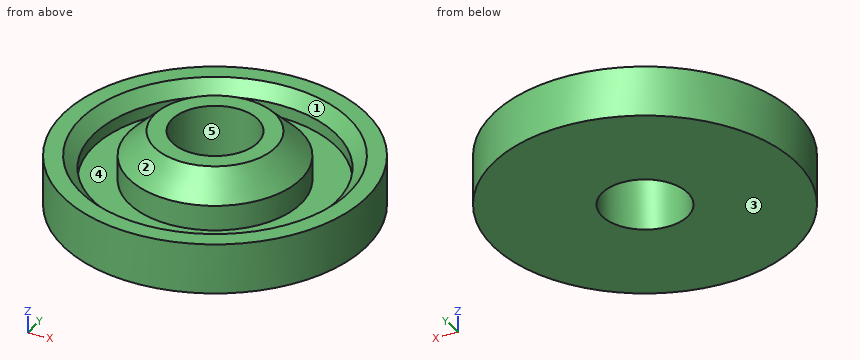
```python
from build123d import *

# Parameters (mm, degrees)
SKETCH2_R          = 1.6933
CUT_EXTRUDE1_DEPTH = 10


with BuildPart() as part:
    # Sketch1 → Revolve1 (revolve)
    with BuildSketch(Plane(origin=(0, 0, 0), x_dir=(1, 0, 0), z_dir=(0, 1, 0)), mode=Mode.PRIVATE) as revolve1_sk:
        Polygon((0, 0), (6, 0), (6, -2), (5.3, -2), (4.8, -1.5), (4.8, -1), (3.4, -1), (3.4, -2), (2.39055, -3), (0, -3), align=None)
    revolve(revolve1_sk.sketch.rotate(Axis((0, 0, 0), (0, 0, 1)), 180), axis=Axis((0, 0, 0), (0, 0, 1)))

    # Sketch2 → Cut-Extrude1 (cut, through all)
    with BuildSketch(Plane.XY.offset(3)):
        Circle(SKETCH2_R)
    extrude(amount=-CUT_EXTRUDE1_DEPTH, mode=Mode.SUBTRACT)


solid = part.part
```
Could you check a few things on this model? Use its own coordinates, in mm. Face numbers are marked on the shaded views. A direction names the side the tool comes from. Round coordinates to 2 decimals unless told otherwise and drop trailing zeros. Order: outer loops, then holes, each group sorted by start corner. A loop starts at its lowest first (then second) coordinate and runs counter-clockwise, first axis right, second up. Notation, with made-up numbers: (-21.5, -2.75) -> (1.5, -2.75) arc R16 cw to (1.5, 6.25) -> close; hole circle Ø11 at (79, 43.25). An arc over 180 degrees is marked (long way). One line per question, with ' | ' between items.
Q1. I'm going to push flat-ended pins straight in: pin 1 (3 mm diameter, centred on x = 0.5, y = -2.5, fed in from +Z); pin 2 (1 mm diameter, centred on y = 4.5, z = 2, fed in from +X). Where does each tip first touch, or does it pass through?
Computed values:
pin 1: z = 3 | pin 2: x = 4.47
Q2. We'd pull the mould along Y, two halves only. Please class the marked faces 1, 2 and 3: released by +Y, released by -Y, zero draft, split by the parting line, or undercut.
Computed values:
face 1: undercut | face 2: split by the parting line | face 3: zero draft
Q3. If we section it at C-C on z = 0.45: Write out the boundary of the cut face in (x, y).
Computed values:
outline: circle Ø12 at (0, 0); hole circle Ø3.39 at (0, 0)
Q4. Which directions (+Z, -Z, +X, -X, +Y, -Y) give clear straight access to the entire face, cutting with the end or side of a thin tool? Please do the marked faces 4 and 5.
Computed values:
face 4: +Z | face 5: +Z, -Z
Q5. If we section it at D-D on z = 2.5: Write out the boundary of the cut face in (x, y), plus the area to 3 significant figures.
Computed values:
outline: circle Ø5.79 at (0, 0); hole circle Ø3.39 at (0, 0) | area: 17.3 mm²
Q6. If we section it at A-A on x = 0: Write out the boundary of the cut face in (y, z), plus the area to 3 significant figures.
Computed values:
outline: (-6, 0) -> (-1.69, 0) -> (-1.69, 3) -> (-2.39, 3) -> (-3.4, 2) -> (-3.4, 1) -> (-4.8, 1) -> (-4.8, 1.5) -> (-5.3, 2) -> (-6, 2) -> close; (1.69, 0) -> (6, 0) -> (6, 2) -> (5.3, 2) -> (4.8, 1.5) -> (4.8, 1) -> (3.4, 1) -> (3.4, 2) -> (2.39, 3) -> (1.69, 3) -> close | area: 16.6 mm²
Q7. If I drill on line 1 (Y direction, x = 0, z = 1.2); line 2 (Y direction, x = 2.5, z = 1.3); line 3 (Y direction, x = 1.25, z = 1.9), over which ranges is the centre line in solid material (lowest first)? Write a range as from..to.
Computed values:
line 1: -6..-4.8, -3.4..-1.69, 1.69..3.4, 4.8..6 | line 2: -5.45..-4.1, -2.3..2.3, 4.1..5.45 | line 3: -5.87..-5.05, -3.16..-1.14, 1.14..3.16, 5.05..5.87
